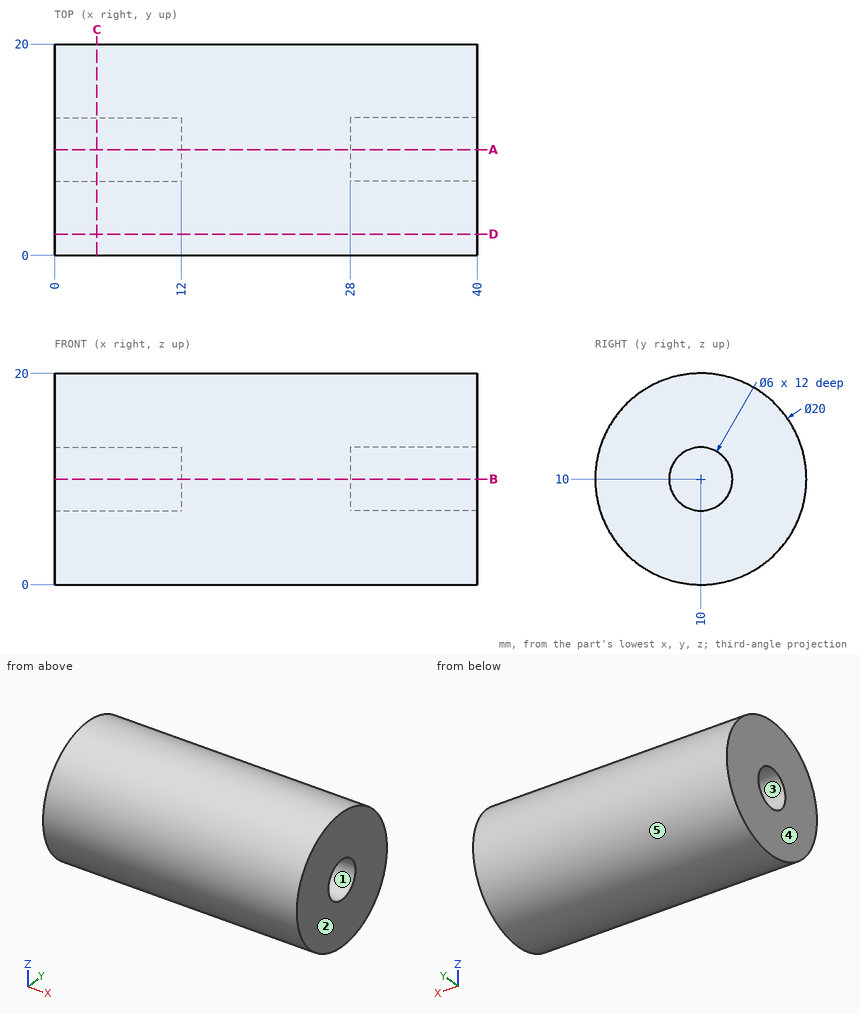
Geometry check sheet. Reference: drawing and pictorial views, mm from the part's lowest x, y, z. A direction names the side the tool comes from. Give positions to 0.01 mm unless a question says otherwise; leave off trailing zeros. Write each loop counter-clockwise with the first axis right and the second up, starting at its lowest first coordinate (ties: lowest second). Pieces come first, ordered by that corner, then holes. Notation, with made-up numbers: M -12,13 L 5,13 A15 ccw 5,35 Z; hole C -18,-30.5 d11. An arc over 180 degrees is marked long. Put each result on its own line as item: value. Start each with the question number.
1. Section check D-D (y = 2). Record the cut outline in (x, z), and give its area (3 significant figures).
2. Go/stop test with flat-tipped pins: pin 1 Ø1 at (x, z) = (4.5, 16.5) entering from +Y; pin 2 Ø5.5 at (y, z) = (10, 10) entering from -X; pin 3 Ø12 at (x, y) = (19, 15) entering from +Z; pin 4 Ø1.8 at (y, z) = (10.5, 8.5) entering from +X. Record where each tip stops, or that it passes through.
3. Section check A-A (y = 10). Record the cut outline in (x, z).
4. Set-up check for the marked faces 1 and 2: record each of +Z, -Z, +X, -X, +Y, -Y from which the full face is reachable in a straight line by a thin tool's end or side.
5. Draft check along Z on the marked faces 3, 4 and 5. Enter one of: +Z half, -Z half, draft (parallel to the pull), parting line (faces both ways), or undercut.
6. Section check C-C (x = 4). Record the cut outline in (y, z).
7. Scan lines: line 1 along Z through (x, y) = (32.75, 10); line 2 along Y through (x, z) = (11.5, 8); line 3 along Y through (x, z) = (36, 8.25). Record each from-to range of solid material in increasing order. Write a range as [from, to].
Answer list:
1. outline: M 0,4 L 40,4 L 40,16 L 0,16 Z
1. area: 480 mm2
2. pin 1: y = 18
2. pin 2: x = 12
2. pin 3: z = 20
2. pin 4: x = 28
3. outline: M 0,0 L 40,0 L 40,7 L 28,7 L 28,13 L 40,13 L 40,20 L 0,20 L 0,13 L 12,13 L 12,7 L 0,7 Z
4. face 1: +X
4. face 2: +Z, -Z, +X, +Y, -Y
5. face 3: undercut
5. face 4: draft
5. face 5: parting line
6. outline: C 10,10 d20; hole C 10,10 d6
7. line 1: [0, 7], [13, 20]
7. line 2: [0.2, 7.76], [12.24, 19.8]
7. line 3: [0.15, 7.56], [12.44, 19.85]
